```python
from build123d import *

# Parameters (mm, degrees)
F0_R     = 6.35
F1_DEPTH = 3.175


with BuildPart() as f1:
    # F0 (on Top) → F1 (new body)
    with BuildSketch(Plane.XY):
        Polygon((152.4, -152.4), (152.4, 292.1), (88.9, 292.1), (-88.9, 292.1), (-152.4, 292.1), (-152.4, -152.4), (-88.9, -215.9), (-12.7, -292.1), (12.7, -292.1), (152.4, -292.1), align=None)
        with BuildLine():
            ThreePointArc((-82.55, -165.1), (-84.409872, -169.590128), (-88.9, -171.45))
            ThreePointArc((-88.9, -171.45), (-93.390128, -169.590128), (-95.25, -165.1))
            ThreePointArc((-95.25, -165.1), (-93.390128, -160.609872), (-88.9, -158.75))
            ThreePointArc((-88.9, -158.75), (-84.409872, -160.609872), (-82.55, -165.1))
        make_face(mode=Mode.SUBTRACT)
        with BuildLine():
            ThreePointArc((88.9, -158.75), (93.390128, -160.609872), (95.25, -165.1))
            ThreePointArc((95.25, -165.1), (93.390128, -169.590128), (88.9, -171.45))
            ThreePointArc((88.9, -171.45), (84.409872, -169.590128), (82.55, -165.1))
            ThreePointArc((82.55, -165.1), (84.409872, -160.609872), (88.9, -158.75))
        make_face(mode=Mode.SUBTRACT)
        with Locations((0, -139.7)):
            Circle(F0_R, mode=Mode.SUBTRACT)
        with BuildLine():
            ThreePointArc((-88.9, 6.35), (-84.409872, 4.490128), (-82.55, 0))
            ThreePointArc((-82.55, 0), (-84.409872, -4.490128), (-88.9, -6.35))
            ThreePointArc((-88.9, -6.35), (-95.25, 0), (-88.9, 6.35))
        make_face(mode=Mode.SUBTRACT)
        with BuildLine():
            ThreePointArc((-88.9, 215.9), (-95.25, 222.25), (-88.9, 228.6))
            ThreePointArc((-88.9, 228.6), (-84.409872, 226.740128), (-82.55, 222.25))
            ThreePointArc((-82.55, 222.25), (-84.409872, 217.759872), (-88.9, 215.9))
        make_face(mode=Mode.SUBTRACT)
        with Locations((0, 120.65)):
            Circle(F0_R, mode=Mode.SUBTRACT)
        with BuildLine():
            ThreePointArc((88.9, 6.35), (93.390128, 4.490128), (95.25, 0))
            ThreePointArc((95.25, 0), (93.390128, -4.490128), (88.9, -6.35))
            ThreePointArc((88.9, -6.35), (82.55, 0), (88.9, 6.35))
        make_face(mode=Mode.SUBTRACT)
        with BuildLine():
            ThreePointArc((88.9, 158.75), (82.55, 165.1), (88.9, 171.45))
            ThreePointArc((88.9, 171.45), (93.390128, 169.590128), (95.25, 165.1))
            ThreePointArc((95.25, 165.1), (93.390128, 160.609872), (88.9, 158.75))
        make_face(mode=Mode.SUBTRACT)
    extrude(amount=F1_DEPTH)


solid = f1.part
```
Read the model definition and answer for the solid it produces. Units are mm, in the model's axes. Give positions to 0.01 mm unless a question says otherwise; leave off trailing zeros. Loops run counter-clockwise (first coordinate to the right, second up) from the corner with the lowest first, then second, coordinate; pieces in that order, holes last.
Item 1: The part is cut by section C-C (z = 0.6). Give the number of separate pieces and of enclosed holes in the cut face, and give its area (3 significant figures).
Item 2: The part is cut by section A-A (y = -139.7). Write down the section's boundary in (x, z) (3 decimals).
Item 3: The mould has two halves that part along Y. Classify faces 1 (the cylindrical face through (-0.827, 126.946, 1.565)), 2 (the cylindrical face through (-1.38, -145.9, 1.57)), 3 (the flat face through (-2, 4, 0)), 4 (the flat face through (-83.5, -221.3, 1.6)): released by +Y, released by -Y, zero draft, split by the parting line, or undercut.
Item 4: Each of these flat-tipped pins is pushed along its axis until it touches: pin 1 Ø11.5 at (x, y) = (0, -139.7) entering from +Z; pin 2 Ø1.5 at (x, z) = (-96, 1.5) entering from -Y. Where does it stop, or does it pass through?
Item 5: Find the intervals of material crossed by line 1 along Y through (x, z) = (0, 1.15); line 2 along Y through (x, z) = (-85, 2.65); line 3 along X through (y, z) = (223.5, 1), in increasing order.
Item 6: The part is cut by section B-B (x = 0). Write down the section's boundary in (y, z) (3 decimals), and give its area (3 significant figures).
Item 7: The part is cut by section D-D (y = -234.5). Write down the section's boundary in (x, z) (3 decimals), and give its area (3 significant figures).
Taken from the geometry:
1. separate pieces: 1
1. enclosed holes: 8
1. area: 167,000 mm2
2. outline: (-152.4, 0) - (-6.35, 0) - (-6.35, 3.175) - (-152.4, 3.175) - close; (6.35, 0) - (152.4, 0) - (152.4, 3.175) - (6.35, 3.175) - close
3. face 1: undercut
3. face 2: undercut
3. face 3: zero draft
3. face 4: released by -Y
4. pin 1: passes through
4. pin 2: stops at y = -209.55
5. line 1: y = -292.1 to -146.05, -133.35 to 114.3, 127 to 292.1
5. line 2: y = -219.8 to -170.11, -160.09 to -5.01, 5.01 to 217.24, 227.26 to 292.1
5. line 3: x = -152.4 to -95.13, -82.67 to 152.4
6. outline: (-292.1, 0) - (-146.05, 0) - (-146.05, 3.175) - (-292.1, 3.175) - close; (-133.35, 0) - (114.3, 0) - (114.3, 3.175) - (-133.35, 3.175) - close; (127, 0) - (292.1, 0) - (292.1, 3.175) - (127, 3.175) - close
6. area: 1,770 mm2
7. outline: (-70.3, 0) - (152.4, 0) - (152.4, 3.175) - (-70.3, 3.175) - close
7. area: 707 mm2
